Work out the finished part from the listing and answer in its coordinate system (mm). Coordinates: 2 decimals unless noted, no trailing zeros. Order: outer loops, then holes, each group sorted by start corner. A loop starts at its lowest first (then second) coordinate and runs counter-clockwise, first axis right, second up. Notation, with made-up numbers: (-9.75, -3.75) -> (47.25, -3.75) arc R18 cw to (47.25, 20.25) -> close; hole circle Ø4 at (85.5, 6.25). An arc over 180 degrees is marked (long way). Write item = value, one per line. Start each with the question number.
Q1. The part is cut by section A-A, the plane x = 10. Determine the outline of the cut face in (y, z), plus the area to 3 significant figures.
Q2. Flat-ended cylindrical pins translate along their axes: pin 1 (8 mm diameter, centred on x = 35, y = -5, fed in from -Z); pin 2 (2 mm diameter, centred on x = 131, y = -4.5, fed in from +Z); pin 3 (5 mm diameter, centred on x = 111, z = 1.5, fed in from +Y). Find the tip coordinate at first contact, or state that the pin passes through.
Q3. Straight lines are drawn through the part: L1, parallel to Z at x = 30, y = 0; L2, parallel to Y at x = 7.5, z = -2; L3, parallel to Z at x = 27.5, y = 0. For each, find the intervals that lie inside material, in ascending order. Write a range as from..to.
```python
from build123d import *

# Parameters (mm, degrees)
F2_R = 2


# Not quite as in the source:
# - a fillet or chamfer that OpenCascade refuses, or shapes differently, is made with other operations: its cross-section is extruded or revolved along the edge and cut away or added


with BuildPart() as f1:
    # F0 (on Front) → F1 (revolve)
    with BuildSketch(Plane.XZ):
        with BuildLine():
            ThreePointArc((-7.0685046336, 10.3095219212), (4.6853520259, 11.5886788028), (12.2474487139, 2.5))
            Line((12.2474487139, 2.5), (74.2474487139, 2.5))
            Line((74.2474487139, 2.5), (149.7373398729, 7.1184875673))
            ThreePointArc((149.7373398729, 7.1184875673), (140.4668689382, 12.5188941968), (130.5825582503, 8.3467933662))
            add(Edge.make_bspline(
                [(13.7809895682, 12.3177978136), (17.1554645129, 6.7528548074), (43.3358067225, 6.5220205059), (122.1384170347, 6.3653155344), (130.5825582503, 8.3467933662)],
                knots=[0, 0, 0, 0, 0.3738465221, 1, 1, 1, 1], degree=3))
            ThreePointArc((13.7809895682, 12.3177978136), (2.4835532955, 18.3159979112), (-10.003236638, 15.5428141988))
            Line((-10.003236638, 15.5428141988), (-7.0685046336, 10.3095219212))
        make_face()
    revolve(axis=Axis((35, 0, 0), (1, 0, 0)))

    # F2
    f2_edges = [f1.edges().sort_by_distance(p)[0] for p in [
        (149.73734, 0, -7.118488),
        (-7.068505, 0, -10.309522),
        (12.247449, 0, -2.5),
    ]]
    fillet(f2_edges, radius=F2_R)

    # F3: fillet of radius 5 on 1 edges, made by hand

    # F3_s1 → F3_t2 (revolve, cut)
    with BuildSketch(Plane.XZ):
        with BuildLine():
            ThreePointArc((74.4000566425, 2.5089358376), (74.2473895925, 2.5019345041), (74.094579917, 2.4996))
            Line((74.094579917, 2.4996), (74.094579917, 1.99936))
            ThreePointArc((74.094579917, 1.99936), (74.1710143155, 1.99976), (74.2474487139, 1.99976))
            Line((74.2474487139, 1.99976), (74.2779963865, 2.0006935838))
            ThreePointArc((74.2779963865, 2.0006935838), (74.3542881375, 2.0053611293), (74.430604315, 2.0096294213))
            Line((74.430604315, 2.0096294213), (74.4000566425, 2.5089358376))
        make_face()
    revolve(axis=Axis((74.2474487139, 0, 0), (1, 0, 0)), mode=Mode.SUBTRACT)


solid = f1.part
```
Model answer:
q1.outline = circle Ø31.09 at (0, 0); hole circle Ø15 at (0, 0)
q1.area = 582 mm2
q2.pin_1 = -6.6
q2.pin_2 = 8.77
q2.pin_3 = 7.05
q3.L1 = -6.84..-2.5, 2.5..6.84
q3.L2 = -16.77..-9.8, 9.8..16.77
q3.L3 = -7..-2.5, 2.5..7
